Here's how the part is built. I have some questions about the finished solid (model axes, mm). A direction names the side the tool comes from. Give positions to 0.01 mm unless a question says otherwise; leave off trailing zeros. Write each loop counter-clockwise with the first axis right and the second up, starting at its lowest first coordinate (ties: lowest second). Pieces come first, ordered by that corner, then holes. Notation, with made-up numbers: (51.5, 69.5) - (97.5, 69.5) arc R32 cw to (97.5, 107.5) - close; hole circle Ø9 at (52, -33.75). An arc over 180 degrees is marked (long way). Write each question's results on one line, items separated by ' | '. Start each with the question number.
Item 1: Suppose I cut it at D-D on z = 18. List the corners of the cut face in (x, y) for me, then the cut area to 3 significant figures.
Item 2: We'd pull the mould along Z, two halves only. Please class faces 4 (the flat face through (38, -13, 0)), 5 (the flat face through (38, -25.4, 13)), 6 (the flat face through (19, -15, 12.7)), 7 (the cylindrical face through (38.278, -6.643, 33.657)): +Z half, -Z half, draft (parallel to the pull), parting line (faces both ways), or undercut.
Item 3: Please list where these lines run through material, in increasing order: line 1 along Y through (x, z) = (12.7, 8.5); line 2 along X through (y, z) = (-12.75, 11); line 3 along X through (y, z) = (-9.5, 24).
Item 4: Will these pins go through, and if not, where does the flat tip stop? P1, Ø6, axis at y = -15.5, z = 15, coming from the -X side; P2, Ø1, axis at x = 37, y = -6.5, coming from the -Z side; P3, Ø12.5, axis at y = -7.5, z = 36, coming from the +X side; P4, Ø12.5, axis at x = 61, y = -7.5, coming from the +Z side.
Item 5: Suppose I cut it at A-A on x = 40.5. List the corners of the cut face in (y, z) for me.
Item 6: Suppose I cut it at C-C on y = -17.5. List the corners of the cut face in (x, z) for me, then the cut area to 3 significant figures.
Item 7: Suppose I cut it at B-B on z = 34.5. List the corners of the cut face in (x, y) for me, then the cut area to 3 significant figures.
Item 8: Which directions (+Z, -Z, +X, -X, +Y, -Y) give clear straight access to the entire face, cutting with the end or side of a thin tool? Please do faces 1 (the cylindrical face through (7.66, -16.56, 6.44)), 2 (the flat face through (25.4, -13, 25)), 3 (the flat face through (50.8, -13, 25)).
```python
from build123d import *

# Parameters (mm, degrees)
F1_DEPTH = 25.4
F2_R     = 6.35
F3_DEPTH = 25.4
F4_R     = 6.35
F5_DEPTH = 25.4
F6_R     = 6.35
F7_DEPTH = 25.4


# Not quite as in the source:
# - ends of sketch curves that miss each other by under 0.0002 mm in the source are joined


with BuildPart() as f1:
    # F0 (on Front) → F1 (new body)
    with BuildSketch(Plane.XZ):
        Polygon((0, 12.7), (0, 0), (76.2, 0), (76.2, 12.7), (50.8, 12.7), (50.8, 44.45), (25.4, 44.45), (25.4, 12.7), align=None)
    extrude(amount=F1_DEPTH)

    # F2 (on face) → F3 (cut)
    with BuildSketch(Plane.YZ.offset(50.8)):
        with BuildLine():
            ThreePointArc((-25.4, 32.294421317), (-22.4820111245, 40.1263057346), (-15.3294772723, 44.45))
            Line((-15.3294772723, 44.45), (-25.4, 44.45))
            Line((-25.4, 44.45), (-25.4, 32.294421317))
        make_face()
        with BuildLine():
            ThreePointArc((-10.0705227277, 44.45), (-2.9179888755, 40.1263057346), (0, 32.294421317))
            Line((0, 32.294421317), (0, 44.45))
            Line((0, 44.45), (-10.0705227277, 44.45))
        make_face()
        with Locations((-12.7, 31.75)):
            Circle(F2_R)
    extrude(amount=-F3_DEPTH, mode=Mode.SUBTRACT)

    # F4 (on face) → F5 (cut)
    with BuildSketch(Plane.XY.offset(12.7)):
        with BuildLine():
            ThreePointArc((63.5, -3.1832e-06), (72.4802600435, -3.7197427535), (76.2000063664, -12.7))
            Line((76.2000063664, -12.7), (76.2, 0))
            Line((76.2, 0), (63.5, -3.1832e-06))
        make_face()
        with BuildLine():
            ThreePointArc((76.2000063664, -12.7), (72.4802600435, -21.6802572465), (63.5, -25.3999968168))
            Line((63.5, -25.3999968168), (76.2, -25.4))
            Line((76.2, -25.4), (76.2000063664, -12.7))
        make_face()
        with Locations((63.5, -12.7)):
            Circle(F4_R)
    extrude(amount=-F5_DEPTH, mode=Mode.SUBTRACT)

    # F6 (on face) → F7 (cut)
    with BuildSketch(Plane.XY.offset(12.7)):
        with Locations((12.7, -12.7)):
            Circle(F6_R)
        with BuildLine():
            ThreePointArc((0, -12.7), (3.7197438789, -3.7197438789), (12.7, 0))
            Line((12.7, 0), (0, 0))
            Line((0, 0), (0, -12.7))
        make_face()
        with BuildLine():
            ThreePointArc((12.7, -25.4), (3.7197438789, -21.6802561211), (0, -12.7))
            Line((0, -12.7), (0, -25.4))
            Line((0, -25.4), (12.7, -25.4))
        make_face()
    extrude(amount=-F7_DEPTH, mode=Mode.SUBTRACT)


solid = f1.part
```
Checked values:
1) outline: (25.4, -25.4) - (50.8, -25.4) - (50.8, 0) - (25.4, 0) - close | area: 645 mm^2
2) face 4: -Z half | face 5: draft | face 6: +Z half | face 7: undercut
3) line 1: y = -25.4 to -19.05, -6.35 to 0 | line 2: x = 0 to 6.35, 19.05 to 57.15, 69.85 to 76.2 | line 3: x = 25.4 to 50.8
4) P1: stops at x = 0.03 | P2: stops at z = 0 | P3: stops at x = 50.8 | P4: stops at z = 12.7
5) outline: (-25.4, 0) - (0, 0) - (0, 32.29) arc R12.7 ccw to (-10.07, 44.45) - (-15.33, 44.45) arc R12.7 ccw to (-25.4, 32.29) - close; hole circle Ø12.7 at (-12.7, 31.75)
6) outline: (0.94, 0) - (8.54, 0) - (8.54, 12.7) - (0.94, 12.7) - close; (16.86, 0) - (59.34, 0) - (59.34, 12.7) - (50.8, 12.7) - (50.8, 27.59) - (25.4, 27.59) - (25.4, 12.7) - (16.86, 12.7) - close; (25.4, 35.91) - (50.8, 35.91) - (50.8, 43.78) - (25.4, 43.78) - close; (67.66, 0) - (75.26, 0) - (75.26, 12.7) - (67.66, 12.7) - close | area: 1,310 mm^2
7) outline: (25.4, -25.16) - (50.8, -25.16) - (50.8, -18.42) - (25.4, -18.42) - close; (25.4, -6.98) - (50.8, -6.98) - (50.8, -0.24) - (25.4, -0.24) - close | area: 342 mm^2
8) face 1: +Z, -Z | face 2: +Z, -X, +Y, -Y | face 3: +Z, +X, +Y, -Y
